Check sheet for the drawn part. Datum: minimum x, y, z corner. Units: mm. A direction names the side the tool comes from. Round coordinates to 2 decimals unless told otherwise and drop trailing zeros. Loops run counter-clockwise (first coordinate to the right, second up) from the corner with the lowest first, then second, coordinate; pieces in that order, holes last. Notation, with made-up numbers: (61, 51) - (67, 51) arc R6 cw to (67, 60) - close; hole circle Ø11 at (-13, 78). An arc over 180 degrees is marked (long way). Use CSV: the item, a comma, the result in double quotes.
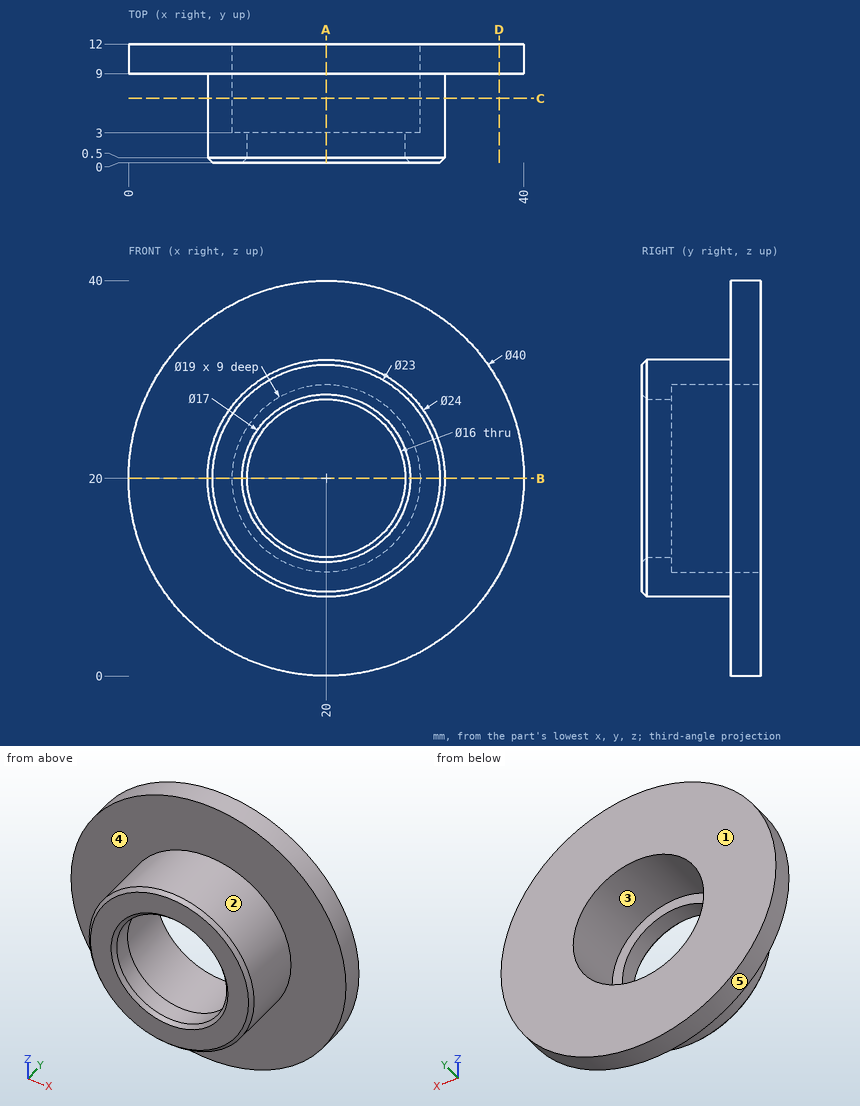
1) Cross-section at C-C, the plane y = 6.5. Record the cut outline in (x, z).
Returned:
outline,"circle Ø24 at (20, 20); hole circle Ø19 at (20, 20)"
2) Cross-section at D-D, the plane x = 37.5. Record the cut outline in (y, z), then the cut area to 3 significant figures.
Returned:
outline,"(9, 10.32) - (12, 10.32) - (12, 29.68) - (9, 29.68) - close"
area,"58.1 mm²"
3) Cross-section at A-A, the plane x = 20. Record the cut outline in (y, z), then the cut area to 4 significant figures.
Returned:
outline,"(0, 8.5) - (0.5, 8) - (9, 8) - (9, 0) - (12, 0) - (12, 10.5) - (3, 10.5) - (3, 12) - (0.5, 12) - (0, 11.5) - close; (0, 28.5) - (0.5, 28) - (3, 28) - (3, 29.5) - (12, 29.5) - (12, 40) - (9, 40) - (9, 32) - (0.5, 32) - (0, 31.5) - close"
area,"116.5 mm²"
4) Cross-section at B-B, the plane z = 20. Record the cut outline in (x, y).
Returned:
outline,"(0, 9) - (8, 9) - (8, 0.5) - (8.5, 0) - (11.5, 0) - (12, 0.5) - (12, 3) - (10.5, 3) - (10.5, 12) - (0, 12) - close; (28, 0.5) - (28.5, 0) - (31.5, 0) - (32, 0.5) - (32, 9) - (40, 9) - (40, 12) - (29.5, 12) - (29.5, 3) - (28, 3) - close"
5) Thickness scan on probe 1 along Z at (x, y) = (20, 7.25); probe 2 along Z at (x, y) = (20, 10.25); probe 3 along X at (y, z) = (1.45, 20). Record the ranges inside material, lowest first. Write a range as [from, to].
Returned:
probe 1,"z = [8, 10.5], [29.5, 32]"
probe 2,"z = [0, 10.5], [29.5, 40]"
probe 3,"x = [8, 12], [28, 32]"
6) Gauge pin test, flat ends, axial feed: pin 1 Ø8 at (x, z) = (11, 28) entering from -Y; pin 2 Ø2 at (x, y) = (31, 8.5) entering from -Z; pin 3 Ø4 at (x, y) = (24, 9) entering from +Z; pin 4 Ø17 at (x, z) = (20, 20) entering from +Y. Record the tip position at first contact, or that the pin passes through.
Returned:
pin 1,"stops at y = 0"
pin 2,"stops at z = 2.76"
pin 3,"stops at z = 39.9"
pin 4,"stops at y = 3"
7) Mould release check, pull along X, two halves, no side actions. Record for the marked faces 1, 2 and 3: +X half, -X half, draft (parallel to the pull), parting line (faces both ways), or undercut.
Returned:
face 1,"draft"
face 2,"parting line"
face 3,"undercut"
8) Access from +Z, -Z, +X, -X, +Y, -Y to the whole of each face (thin tool, end or side, straight path). Record for the marked faces 4 and 5.
Returned:
face 4,"-Y"
face 5,"+Y, -Y"
